Check sheet for the drawn part. Datum: minimum x, y, z corner. Units: mm. A direction names the side the tool comes from. Give positions to 0.01 mm unless a question says otherwise; leave off trailing zeros. Write each loop counter-clockwise with the first axis right and the second up, starting at its lowest first coordinate (ties: lowest second). Pieces come first, ordered by that corner, then holes. Notation, with made-up numbers: (-26, -21) -> (-5, -21) arc R14 cw to (-5, -11) -> close; hole circle Ø6 at (27, 25). An arc over 180 degrees is marked (long way). Write item = value, one per line. Start each with the question number.
1. Depth check by flat-ended pin: P1, Ø2, axis at y = 68.5, z = 43, coming from the +X side; P2, Ø6, axis at x = 38, z = 36.5, coming from the -Y side. Enter the tip coordinate at first touch or a pass-through.
2. Cross-section at A-A, the plane y = 33.5. Record the cut outline in (x, z).
3. Set-up check for the marked faces 1 and 2: record each of +Z, -Z, +X, -X, +Y, -Y from which the full face is reachable in a straight line by a thin tool's end or side.
4. Cross-section at B-B, the plane x = 20. Record the cut outline in (y, z), plus the area to 3 significant figures.
5. Cross-section at C-C, the plane z = 40. Record the cut outline in (x, y).
6. Thickness scan on line 1 along Z through (x, y) = (20, 86); line 2 along Y through (x, z) = (1.65, 40); line 3 along X through (y, z) = (85.7, 20). Record the ranges inside material, lowest first.
7. Cross-section at D-D, the plane z = 73. Record the cut outline in (x, y), plus the area to 3 significant figures.
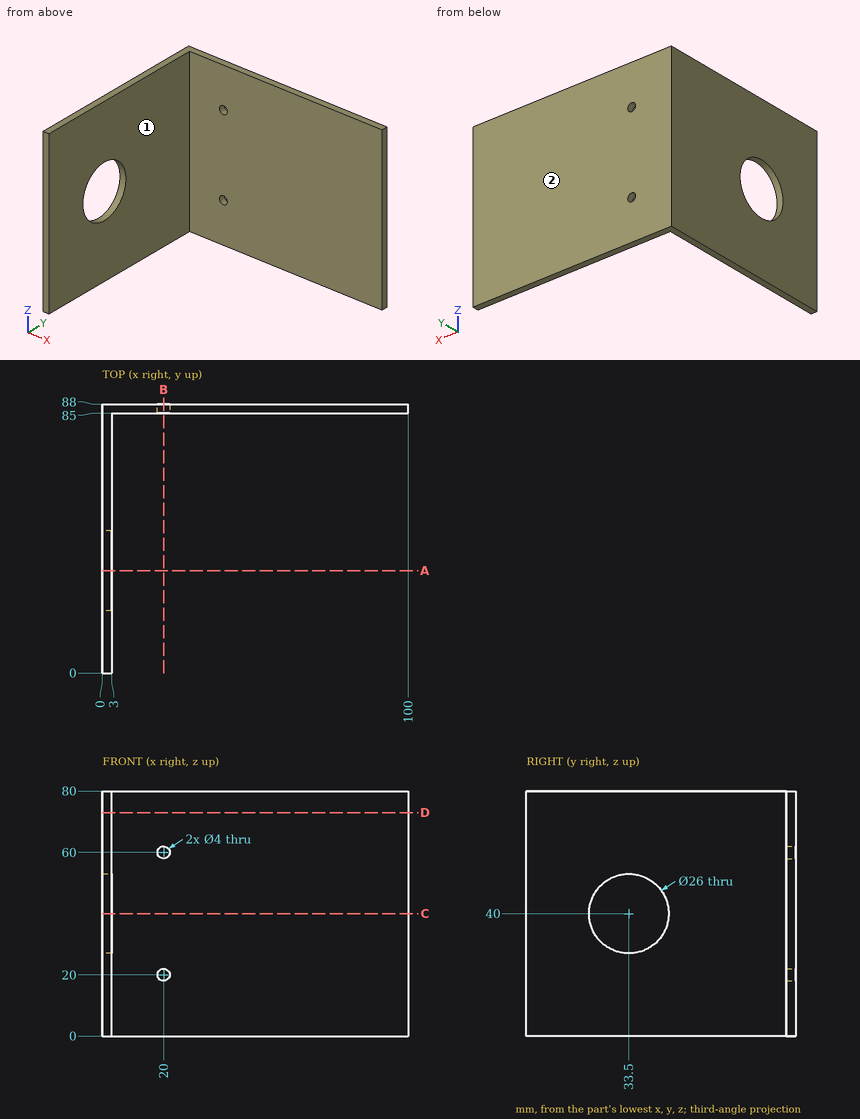
Answers:
q1.P1 = 3
q1.P2 = 85
q2.outline = (0, 0) -> (3, 0) -> (3, 27) -> (0, 27) -> close; (0, 53) -> (3, 53) -> (3, 80) -> (0, 80) -> close
q3.face_1 = +Z, -Z, +X, -Y
q3.face_2 = +Z, -Z, +X, -X, +Y
q4.outline = (85, 0) -> (88, 0) -> (88, 18) -> (85, 18) -> close; (85, 22) -> (88, 22) -> (88, 58) -> (85, 58) -> close; (85, 62) -> (88, 62) -> (88, 80) -> (85, 80) -> close
q4.area = 216 mm^2
q5.outline = (0, 0) -> (3, 0) -> (3, 20.5) -> (0, 20.5) -> close; (0, 46.5) -> (3, 46.5) -> (3, 85) -> (100, 85) -> (100, 88) -> (0, 88) -> close
q6.line_1 = 0 to 18, 22 to 58, 62 to 80
q6.line_2 = 0 to 20.5, 46.5 to 88
q6.line_3 = 0 to 18, 22 to 100
q7.outline = (0, 0) -> (3, 0) -> (3, 85) -> (100, 85) -> (100, 88) -> (0, 88) -> close
q7.area = 555 mm^2
